```python
from build123d import *

# Parameters (mm, degrees)
F0_R     = 3.96875
F0_R_2   = 6.35
F0_W     = 115.8875
F0_H     = 180.975
F1_DEPTH = 6.35
F2_R     = 5.08


with BuildPart() as f1:
    # F0 (on Front) → F1 (new body)
    with BuildSketch(Plane.XZ):
        with BuildLine():
            Line((-44.45, 109.5375), (-69.05625, 109.5375))
            ThreePointArc((-69.05625, 109.5375), (-74.66891, 107.21266), (-76.99375, 101.6))
            Line((-76.99375, 101.6), (-76.99375, 17.4625))
            Line((-76.99375, 17.4625), (-89.69375, 17.4625))
            ThreePointArc((-89.69375, 17.4625), (-98.674006, 13.742756), (-102.39375, 4.7625))
            Line((-102.39375, 4.7625), (-102.39375, -46.0375))
            ThreePointArc((-102.39375, -46.0375), (-98.674006, -55.017756), (-89.69375, -58.7375))
            Line((-89.69375, -58.7375), (-76.99375, -58.7375))
            Line((-76.99375, -58.7375), (-76.99375, -101.6))
            ThreePointArc((-76.99375, -101.6), (-74.66891, -107.21266), (-69.05625, -109.5375))
            Line((-69.05625, -109.5375), (69.05625, -109.5375))
            ThreePointArc((69.05625, -109.5375), (74.66891, -107.21266), (76.99375, -101.6))
            Line((76.99375, -101.6), (76.99375, -58.7375))
            Line((76.99375, -58.7375), (89.69375, -58.7375))
            ThreePointArc((89.69375, -58.7375), (98.674006, -55.017756), (102.39375, -46.0375))
            Line((102.39375, -46.0375), (102.39375, 4.7625))
            ThreePointArc((102.39375, 4.7625), (98.674006, 13.742756), (89.69375, 17.4625))
            Line((89.69375, 17.4625), (76.99375, 17.4625))
            Line((76.99375, 17.4625), (76.99375, 101.6))
            ThreePointArc((76.99375, 101.6), (74.66891, 107.21266), (69.05625, 109.5375))
            Line((69.05625, 109.5375), (44.45, 109.5375))
            ThreePointArc((44.45, 109.5375), (39.959872, 111.397372), (38.1, 115.8875))
            Line((38.1, 115.8875), (38.1, 122.2375))
            ThreePointArc((38.1, 122.2375), (34.380256, 131.217756), (25.4, 134.9375))
            Line((25.4, 134.9375), (-25.4, 134.9375))
            ThreePointArc((-25.4, 134.9375), (-34.380256, 131.217756), (-38.1, 122.2375))
            Line((-38.1, 122.2375), (-38.1, 115.8875))
            ThreePointArc((-38.1, 115.8875), (-39.959872, 111.397372), (-44.45, 109.5375))
        make_face()
        with Locations((-69.05625, -101.6)):
            Circle(F0_R, mode=Mode.SUBTRACT)
        with Locations((-89.69375, -46.0375)):
            Circle(F0_R_2, mode=Mode.SUBTRACT)
        with Locations((-89.69375, 4.7625)):
            Circle(F0_R_2, mode=Mode.SUBTRACT)
        with Locations((69.05625, -101.6)):
            Circle(F0_R, mode=Mode.SUBTRACT)
        Rectangle(F0_W, F0_H, mode=Mode.SUBTRACT)
        with Locations((89.69375, -46.0375)):
            Circle(F0_R_2, mode=Mode.SUBTRACT)
        with Locations((89.69375, 4.7625)):
            Circle(F0_R_2, mode=Mode.SUBTRACT)
        with Locations((-69.05625, 101.6)):
            Circle(F0_R, mode=Mode.SUBTRACT)
        with Locations((-25.4, 122.2375)):
            Circle(F0_R_2, mode=Mode.SUBTRACT)
        with Locations((25.4, 122.2375)):
            Circle(F0_R_2, mode=Mode.SUBTRACT)
        with Locations((69.05625, 101.6)):
            Circle(F0_R, mode=Mode.SUBTRACT)
    extrude(amount=F1_DEPTH)

    # F2
    f2_edges = [f1.edges().sort_by_distance(p)[0] for p in [
        (-57.94375, -3.175, 90.4875),
        (57.94375, -3.175, 90.4875),
        (57.94375, -3.175, -90.4875),
        (-57.94375, -3.175, -90.4875),
    ]]
    fillet(f2_edges, radius=F2_R)


solid = f1.part
```
Design review of the part built by this model. Coordinates are the model's own, in mm. A direction names the side the tool comes from. Coordinates: 2 decimals unless noted, no trailing zeros. Write each loop counter-clockwise with the first axis right and the second up, starting at its lowest first coordinate (ties: lowest second). Pieces come first, ordered by that corner, then holes. Notation, with made-up numbers: M -4,29.25 L 43,29.25 A19 cw 43,52.25 Z; hole C 87.5,30 d10. An arc over 180 degrees is marked long. Answer as a JSON object with one key per item and string values.
Item 1: Add section C-C, the plane y = -4.75. State how many separate pieces and enclosed holes the cut face has, and give its area (3 significant figures).
Outcome:
{"separate pieces": "1", "enclosed holes": "11", "area": "17,400 mm²"}
Item 2: Add section B-B, the plane z = -71.5. Give the boundary of the cut face in (x, y).
Outcome:
{"outline": "M -76.99,-6.35 L -57.94,-6.35 L -57.94,0 L -76.99,0 Z; M 57.94,-6.35 L 76.99,-6.35 L 76.99,0 L 57.94,0 Z"}
Item 3: Wall thickness on probe 1 along Z at (x, y) = (-25.4, -3); probe 2 along Z at (x, y) = (9.5, -0.75); probe 3 along X at (y, z) = (-5.25, -70.5): over which ranges is each line inside the solid? List them lowest first.
Outcome:
{"probe 1": "-109.54 to -90.49, 90.49 to 115.89, 128.59 to 134.94", "probe 2": "-109.54 to -90.49, 90.49 to 134.94", "probe 3": "-76.99 to -57.94, 57.94 to 76.99"}
Item 4: Insertion check: pin 1 Ø1.9 at (y, z) = (-3, 40.5) entering from +X; pin 2 Ø3 at (y, z) = (-2, -76.5) entering from -X; pin 3 Ø7 at (x, z) = (-69.06, 101.6) entering from -Y; pin 4 Ø3 at (x, y) = (-53.5, -3.5) entering from +Z. Each pin has a flat end and moves straight along its axis. Give the tip position at first contact, or say it passes through.
Outcome:
{"pin 1": "x = 76.99", "pin 2": "x = -76.99", "pin 3": "through", "pin 4": "z = 109.54"}
Item 5: Machinability: for faces 4 (the flat face through (-57, -3, 109.538)), 5 (the flat face through (-83, -3, -58.738)), 6 (the flat face through (83, -3, -58.738)), 7 (the cylindrical face through (-56.416, -3.219, -89.039)), which of the approach directions +Z, -Z, +X, -X, +Y, -Y give a long, thin tool a straight path to every point of the face, cutting with its end or side? Answer none if there is none.
Outcome:
{"face 4": "+Z, -X, +Y, -Y", "face 5": "-Z, -X, +Y, -Y", "face 6": "-Z, +X, +Y, -Y", "face 7": "+Y, -Y"}
Item 6: Draft analysis for pull direction X (two halves, no side actions). For faces 1 (the cylindrical face through (-69.917, -3.131, -105.474)), 2 (the flat face through (-1, -3, -109.538)), 3 (the flat face through (38.1, -3, 119)), state which applies: pulls with the +X half, pulls with the -X half, needs draft (parallel to the pull), parting line crosses it, or undercut.
Outcome:
{"face 1": "undercut", "face 2": "needs draft", "face 3": "pulls with the +X half"}
Item 7: Add section A-A, the plane x = 1. Give the boundary of the cut face in (y, z), and give its area (3 significant figures).
Outcome:
{"outline": "M -6.35,-109.54 L 0,-109.54 L 0,-90.49 L -6.35,-90.49 Z; M -6.35,90.49 L 0,90.49 L 0,134.94 L -6.35,134.94 Z", "area": "403 mm²"}
